The model under review builds one solid part; all positions refer to its coordinate system, in mm. A direction names the side the tool comes from. Round coordinates to 2 decimals unless told otherwise and drop trailing zeros. Write each loop counter-clockwise with the first axis right and the second up, starting at its lowest first coordinate (ties: lowest second). Pieces come first, ordered by that corner, then holes. Notation, with made-up numbers: (55.25, 7) - (103.25, 7) arc R32 ccw to (103.25, 46) - close; hole circle Ø9 at (74.5, 89). An arc over 180 degrees is marked (long way). Return JSON: item names as keys, results as strings.
from build123d import *

# Parameters (mm, degrees)
F2_W     = 0.5
F2_H     = 0.5
F3_DEPTH = 9
F4_R     = 1
F5_R     = 1


with BuildPart() as f1:
    # F0 (on Front) → F1 (revolve)
    with BuildSketch(Plane.XZ):
        Polygon((7.75, 0), (9.75, 0), (10.5, 8), (8.5, 8), (8.0775014419, 3.4933487132), (3.35, 3.4933487132), (3.35, 10), (4, 10), (2, 13), (0, 13), (0, 8), (0, 1.4933487132), (3.25, 1.4933487132), (7.75, 1.5), align=None)
    revolve(axis=Axis((0, 0, 4), (0, 0, 1)))

    # F2 (on face) → F3 (cut)
    with BuildSketch(Plane.XY.offset(13)):
        with BuildLine():
            ThreePointArc((-1.9843134833, -0.25), (-2, 0), (-1.9843134833, 0.25))
            Line((-1.9843134833, 0.25), (-4, 0.25))
            Line((-4, 0.25), (-4, -0.25))
            Line((-4, -0.25), (-1.9843134833, -0.25))
        make_face()
        with BuildLine():
            Line((-0.25, -0.25), (-0.25, 0.25))
            Line((-0.25, 0.25), (-1.9843134833, 0.25))
            ThreePointArc((-1.9843134833, 0.25), (-2, 0), (-1.9843134833, -0.25))
            Line((-1.9843134833, -0.25), (-0.25, -0.25))
        make_face()
        Rectangle(F2_W, F2_H)
        with BuildLine():
            Line((1.9843134833, 0.25), (0.25, 0.25))
            Line((0.25, 0.25), (0.25, -0.25))
            Line((0.25, -0.25), (1.9843134833, -0.25))
            ThreePointArc((1.9843134833, -0.25), (1.9960745185, -0.1252458251), (2, 0))
            ThreePointArc((2, 0), (1.9960745185, 0.1252458251), (1.9843134833, 0.25))
        make_face()
        with BuildLine():
            Line((4, 0.25), (1.9843134833, 0.25))
            ThreePointArc((1.9843134833, 0.25), (1.9960745185, 0.1252458251), (2, 0))
            ThreePointArc((2, 0), (1.9960745185, -0.1252458251), (1.9843134833, -0.25))
            Line((1.9843134833, -0.25), (4, -0.25))
            Line((4, -0.25), (4, 0.25))
        make_face()
        with BuildLine():
            Line((0.25, 1.9843134833), (0.25, 4))
            Line((0.25, 4), (-0.25, 4))
            Line((-0.25, 4), (-0.25, 1.9843134833))
            ThreePointArc((-0.25, 1.9843134833), (0, 2), (0.25, 1.9843134833))
        make_face()
        with BuildLine():
            Line((0.25, 0.25), (0.25, 1.9843134833))
            ThreePointArc((0.25, 1.9843134833), (0, 2), (-0.25, 1.9843134833))
            Line((-0.25, 1.9843134833), (-0.25, 0.25))
            Line((-0.25, 0.25), (0.25, 0.25))
        make_face()
        with BuildLine():
            Line((0.25, -1.9843134833), (0.25, -0.25))
            Line((0.25, -0.25), (-0.25, -0.25))
            Line((-0.25, -0.25), (-0.25, -1.9843134833))
            ThreePointArc((-0.25, -1.9843134833), (0, -2), (0.25, -1.9843134833))
        make_face()
        with BuildLine():
            Line((0.25, -4), (0.25, -1.9843134833))
            ThreePointArc((0.25, -1.9843134833), (0, -2), (-0.25, -1.9843134833))
            Line((-0.25, -1.9843134833), (-0.25, -4))
            Line((-0.25, -4), (0.25, -4))
        make_face()
    extrude(amount=-F3_DEPTH, mode=Mode.SUBTRACT)

    # F4
    f4_edges = [f1.edges().sort_by_distance(p)[0] for p in [
        (-9.75, 0, 0),
    ]]
    fillet(f4_edges, radius=F4_R)

    # F5
    f5_edges = [f1.edges().sort_by_distance(p)[0] for p in [
        (-1.414214, -1.414214, 13),
        (1.414214, -1.414214, 13),
        (1.414214, 1.414214, 13),
        (-1.414214, 1.414214, 13),
    ]]
    fillet(f5_edges, radius=F5_R)


solid = f1.part
(1) Clearance check with flat-ended pins moving along their axes: pin 1 Ø3 at (y, z) = (2, 8.5) entering from +X; pin 2 Ø1.9 at (x, y) = (1, -2.5) entering from -Z; pin 3 Ø1.1 at (y, z) = (2.5, 8) entering from -X. State where each tip first meets the part, or that it passes through.
Filled in:
{"pin 1": "stops at x = 10.48", "pin 2": "stops at z = 1.49", "pin 3": "stops at x = -10.32"}
(2) Wall thickness on line 1 (Z direction, x = -7, y = 1.5); line 2 (Z direction, x = -6, y = -5); line 3 (Y direction, x = 0, z = 1.1): over which ranges is each line inside the solid? List them lowest first.
Filled in:
{"line 1": "z = 1.5 to 3.49", "line 2": "z = 0 to 3.49", "line 3": "y = -9.85 to -7.75, 7.75 to 9.85"}
(3) For faces 4 (the flat face through (-0.25, -2, 9)), 5 (the cylindrical face through (-1.009, 7.684, 0.74)), 6 (the flat face through (-3, 2, 10)), list the 3-axis set-ups (+Z, -Z, +X, -X, +Y, -Y) from which the entire face can be reached by the end or side of a thin tool; tool diameter is ignored.
Filled in:
{"face 4": "+Z", "face 5": "-Z", "face 6": "-X, +Y"}
(4) Add section A-A (z = 7.5). Write out the cut boundary in (x, y).
Filled in:
{"outline": "circle Ø20.91 at (0, 0); (-3.34, -0.25) arc R3.35 ccw to (-0.25, -3.34) - (-0.25, -0.25) - close; (-3.34, 0.25) - (-0.25, 0.25) - (-0.25, 3.34) arc R3.35 ccw to start; (0.25, -3.34) arc R3.35 ccw to (3.34, -0.25) - (0.25, -0.25) - close; (0.25, 0.25) - (3.34, 0.25) arc R3.35 ccw to (0.25, 3.34) - close; hole circle Ø16.91 at (0, 0)"}
(5) Mouldability with a two-part tool opening along Z and no side actions: class faces 1 (the flat face through (3, 2, 10)), 2 (the flat face through (0.25, -2, 9)), 3 (the conical face through (-2.24, -2.195, 11.295)) as released by +Z, released by -Z, zero draft, split by the parting line, or undercut.
Filled in:
{"face 1": "undercut", "face 2": "zero draft", "face 3": "released by +Z"}
